from build123d import *

# Parameters (mm, degrees)
ESQUISSE1_R             = 1.5
EXTRUSION1_DEPTH        = 5
ESQUISSE2_R             = 2.9
ENL_V_MAT_EXTRU_1_DEPTH = 71.807414866
ESQUISSE3_R             = 2.1
ENL_V_MAT_EXTRU_2_DEPTH = 71.887234394


with BuildPart() as part:
    # Esquisse1 → Extrusion1 (new body)
    with BuildSketch(Plane.XY):
        with BuildLine():
            Line((-60, 10), (60, 10))
            ThreePointArc((60, 10), (70, 0), (60, -10))
            Line((60, -10), (-60, -10))
            ThreePointArc((-60, -10), (-70, 0), (-60, 10))
        make_face()
        with Locations((-40, 0)):
            Circle(ESQUISSE1_R, mode=Mode.SUBTRACT)
        with Locations((-20, 0)):
            Circle(ESQUISSE1_R, mode=Mode.SUBTRACT)
        with Locations((-60, 0)):
            Circle(ESQUISSE1_R, mode=Mode.SUBTRACT)
        with Locations((60, 0)):
            Circle(ESQUISSE1_R, mode=Mode.SUBTRACT)
    extrude(amount=EXTRUSION1_DEPTH)

    # Esquisse2 → Enlèv. mat.-Extru.1 (cut, through all)
    with BuildSketch(Plane(origin=(0, 0, 1.3), x_dir=(-1, 0, 0), z_dir=(0, 0, -1))):
        with Locations((-60, 0)):
            Circle(ESQUISSE2_R)
        with Locations((60, 0)):
            Circle(ESQUISSE2_R)
        with Locations((20, 0)):
            Circle(ESQUISSE2_R)
        with Locations((40, 0)):
            Circle(ESQUISSE2_R)
    extrude(amount=-ENL_V_MAT_EXTRU_1_DEPTH, mode=Mode.SUBTRACT)

    # Esquisse3 → Enlèv. mat.-Extru.2 (cut, through all)
    with BuildSketch(Plane(origin=(0, 0, 0), x_dir=(-1, 0, 0), z_dir=(0, 0, -1))):
        with Locations((-6, 0)):
            Circle(ESQUISSE3_R)
        with Locations((-33, 0)):
            Circle(ESQUISSE3_R)
    extrude(amount=-ENL_V_MAT_EXTRU_2_DEPTH, mode=Mode.SUBTRACT)


solid = part.part
Geometry check sheet. Reference: the model listing, model coordinates, mm. A direction names the side the tool comes from. Round coordinates to 2 decimals unless told otherwise and drop trailing zeros. Loops run counter-clockwise (first coordinate to the right, second up) from the corner with the lowest first, then second, coordinate; pieces in that order, holes last.
Item 1: Cross-section at B-B on y = 0. Count the separate pieces of the cut face and the enclosed holes in it, then the cut area to 3 significant figures.
Item 2: Access from +Z, -Z, +X, -X, +Y, -Y to the whole of each face (thin tool, end or side, straight path). Record for faces 4 (the flat face through (-21.2, -1.2, 1.3)), 5 (the cylindrical face through (61.43, 0.45, 0.64)).
Item 3: Cross-section at C-C on z = 2.15. Record the boundary of the cut face in (x, y), then the cut area to 3 significant figures.
Item 4: Thickness scan on line 1 (Y direction, x = -22, z = 3.1); line 2 (Y direction, x = 59.5, z = 4.3); line 3 (X direction, y = -4.5, z = 2.5). Record the ranges inside material, lowest first.
Item 5: Gauge pin test, flat end, axial feed: pin 1 (3.5 mm diameter, centred on x = 60, y = 0, fed in from +Z). Record the tip position at first contact, or that the pin passes through.
Item 6: Cross-section at A-A on x = 33. Record the boundary of the cut face in (y, z).
Item 7: Mould release check, pull along Y, two halves, no side actions. Record for faces 1 (the cylindrical face through (70, 0, 2)), 2 (the cylindrical face through (-42.766, 0.871, 3.124)), 3 (the flat face through (-1, 10, 2)): pulls with the +Y half, pulls with the -Y half, needs draft (parallel to the pull), parting line crosses it, or undercut.
Item 8: Cross-section at D-D on x = -40. Record the boundary of the cut face in (y, z).
Answer sheet:
1. separate pieces: 7
1. enclosed holes: 0
1. area: 557 mm2
2. face 4: +Z
2. face 5: +Z, -Z
3. outline: (-60, -10) - (60, -10) arc R10 ccw to (60, 10) - (-60, 10) arc R10 ccw to start; hole circle Ø5.8 at (-60, 0); hole circle Ø5.8 at (-40, 0); hole circle Ø5.8 at (-20, 0); hole circle Ø4.2 at (6, 0); hole circle Ø4.2 at (33, 0); hole circle Ø5.8 at (60, 0)
3. area: 2,580 mm2
4. line 1: y = -10 to -2.1, 2.1 to 10
4. line 2: y = -10 to -2.86, 2.86 to 10
4. line 3: x = -68.93 to 68.93
5. pin 1: stops at z = 1.3
6. outline: (-10, 0) - (-2.1, 0) - (-2.1, 5) - (-10, 5) - close; (2.1, 0) - (10, 0) - (10, 5) - (2.1, 5) - close
7. face 1: parting line crosses it
7. face 2: undercut
7. face 3: pulls with the +Y half
8. outline: (-10, 0) - (-1.5, 0) - (-1.5, 1.3) - (-2.9, 1.3) - (-2.9, 5) - (-10, 5) - close; (1.5, 0) - (10, 0) - (10, 5) - (2.9, 5) - (2.9, 1.3) - (1.5, 1.3) - close
